Source: CAD feature listing. Evaluate the final solid. Frame: model axes, mm. Face numbers are marked on the shaded views. A direction names the side the tool comes from. Coordinates: 2 decimals unless noted, no trailing zeros. Order: outer loops, then holes, each group sorted by start corner. A loop starts at its lowest first (then second) coordinate and runs counter-clockwise, first axis right, second up.
Item 1: Ray query, line 1 (Z direction, x = -3.7, y = 0); line 2 (X direction, y = -1, z = -1.5); line 3 (Z direction, x = -1.75, y = -2). Return the intervals inside material, ascending.
Item 2: Mould query, pull axis Y, two halves, no side actions, for the marked faces 4, 5 and 6. Classes: released by +Y, released by -Y, zero draft, split by the parting line, or undercut.
Item 3: Reachability of the marked faces 1, 2 and 3 from +Z, -Z, +X, -X, +Y, -Y: full face, straight path, thin tool, end or side. Return the list, or none.
Item 4: Section A-A on x = 12. Return the cut outline in (y, z), then the cut area to 3 significant figures.
Item 5: Contact query for flat-ended pins moving along their axis: P1, Ø1, axis at x = 13.5, y = 1.5, coming from the +Z side; P2, Ø3, axis at x = -1, y = -1, coming from the -Z side; P3, Ø1.5, axis at x = 12, z = 1, coming from the -Y side; P4, Ø5, axis at x = -1, y = -3.5, coming from the -Z side. Output: stop coordinate, or through.
Autodesk Inventor part; units mm, degrees
ref_plane "IDS_WORKPLANE{1}" through (-3.8354, 0, 0) normal (-1, 0, 0) x (0, 0, -1)
ref_plane "Work Plane3" through (7, 0, 0) normal (0, 0, -1) x (1, 0, 0)
ref_plane "YZ Plane" through (0, 0, 0) normal (1, 0, 0) x (0, 1, 0)
sketch "Sketch1" plane through (0, 0, 0) normal (0, 0, 1) x (1, 0, 0)
  line L0 (-0.7874, 5.2578) -> (-0.7874, 0)
  line L1 (-0.7874, 0) -> (19.05, 0)
  line L2 (19.05, 0) -> (19.05, 2.413)
  line L3 (19.05, 2.413) -> (0, 2.413)
  line L4 (0, 2.413) -> (0, 5.2578)
  line L5 (-4.7549, 0) -> (23.0175, 0)
  line L6 (0, -1.0516) -> (0, 6.3094)
  line L7 (0, 5.2578) -> (-0.7874, 5.2578)
  dimension "d1" = 0.7874
  dimension "d2" = 4.826
  dimension "d3" = 19.05
  dimension "d22" = 10.5156
revolve "Body" add sketch "Sketch1" angle 360 about axis through (-0.7874, 0, 0) along (1, 0, 0)
sketch "Sketch2" plane through (-0.7874, 0, 0) normal (-1, 0, 0) x (0, 0, 1)
  line L0 (0, 4.5754) -> (3.9624, 2.2877)
  line L1 (3.9624, 2.2877) -> (3.9624, -2.2877)
  line L2 (3.9624, -2.2877) -> (0, -4.5754)
  line L3 (0, -4.5754) -> (-3.9624, -2.2877)
  line L4 (-3.9624, -2.2877) -> (-3.9624, 2.2877)
  line L5 (-3.9624, 2.2877) -> (0, 4.5754)
  circle A0 centre (0, 0) radius 5.2578
  dimension "d11" = 7.9248
extrude "Head" add sketch "Sketch2" along normal blind 3.048 contours L0 L1 L2 L3 L4 L5
ref_plane "IDS_WORKPLANE{1}" through (-3.8354, 0, 0) normal (-1, 0, 0) x (0, 0, -1)
sketch "Sketch3" plane through (-3.8354, 0, 0) normal (-1, 0, 0) x (0, 0, -1)
  circle A0 centre (0, 0) radius 3.1699
  point P0 (0, 0)
  dimension "d15" = 6.3398
extrude "Indent" cut sketch "Sketch3" against normal blind 0.3048
thread "Thread"
sketch "Sketch4" plane through (0, 0, 0) normal (0, 0, 1) x (1, 0, 0)
  line L0 (-3.8354, 3.9624) -> (-3.8354, 4.5754)
  line L1 (-3.8354, 4.5754) -> (-3.3472, 4.5754)
  line L2 (-3.8354, 4.5754) -> (-3.8354, 2.2877)
  line L3 (-4.9666, 0) -> (2.8908, 0)
  line L4 (-0.7874, 4.5754) -> (-3.8354, 4.5754)
  arc A0 (-3.3472, 4.5754) -> (-3.8354, 3.9624) centre (1.7683, 0) ccw
  dimension "d21" = 7.9248
  dimension "d23" = 6.8631
revolve "Chamfer1" cut sketch "Sketch4" angle 360 about axis through (-10, 0, 0) along (1, 0, 0)
chamfer "Chamfer2" distance 0.5334 distance2 3.7084 1 edges at (19.05, -2.413, 0) measured on face at (19.05, -0.4641, 1.0929)
ref_plane "Work Plane3" through (7, 0, 0) normal (0, 0, -1) x (1, 0, 0)
equation "\"d11\" = SW"
equation "\"d12\" = KOH"
equation "\"d15\" = SD3"
equation "\"d16\" = SB"
equation "\"d6\" = GEL"
equation "\"d19\" = -0.5 * GD2 + 0.5 * NND"
equation "\"d20\" = SPTZ"
equation "\"d1\" = SD"
equation "\"d2\" = NND"
equation "\"d3\" = NLG"
equation "\"d22\" = SD2"
equation "\"d21\" = SW"
equation "\"d23\" = 0.866025 * SW"
equation "\"NLG\" = 19.05"
equation "\"NND\" = 4.826"
equation "\"KOH\" = 3.048"
equation "\"GEL\" = 19.05"
equation "\"SW\" = 7.9248"
equation "\"GD2\" = 3.7592"
equation "\"SPTZ\" = 3.7084"
equation "\"SD3\" = 0.8 * SW"
equation "\"SB\" = 0.1 * KOH"
equation "\"SD2\" = 10.5156"
equation "\"SD\" = 0.7874"
equation "\"GD1\" = 3.7592"
equation "\"THREADDIA\" = 4.826"
equation "\"TOA\" = 30deg"
equation "\"E0\" = 9.15077"
properties part number "am-1165" material "Steel, Mild"
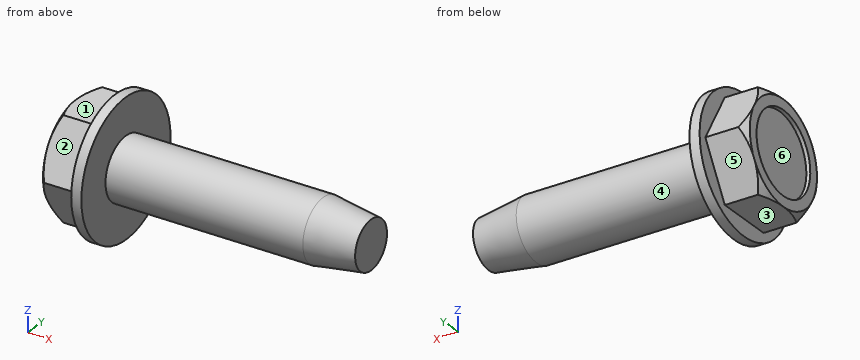
Answer list:
1. line 1: z = -3.96 to -3.17, 3.17 to 3.96
1. line 2: x = -3.53 to 19.05
1. line 3: z = -3.96 to 3.96
2. face 4: split by the parting line
2. face 5: released by +Y
2. face 6: undercut
3. face 1: +Z, -X, +Y, -Y
3. face 2: +Z, -X, -Y
3. face 3: -Z, -X, +Y, -Y
4. outline: circle Ø4.83 at (0, 0)
4. area: 18.3 mm2
5. P1: stops at z = 2.2
5. P2: stops at z = -5.26
5. P3: stops at y = -2.4
5. P4: stops at z = -5.16
